Could you check a few things on this model? Use its own coordinates, in mm. Face numbers are marked on the shaded views. A direction names the side the tool comes from. Round coordinates to 2 decimals unless told otherwise and drop trailing zeros. Loops run counter-clockwise (first coordinate to the right, second up) from the corner with the lowest first, then second, coordinate; pieces in that order, holes last. Notation, with made-up numbers: (-35.5, -30) -> (-25.5, -30) arc R14 cw to (-25.5, -12) -> close; hole circle Ø1 at (-23, 22). An arc over 180 degrees is marked (long way). Write each question's results on one line, items separated by ' | '.
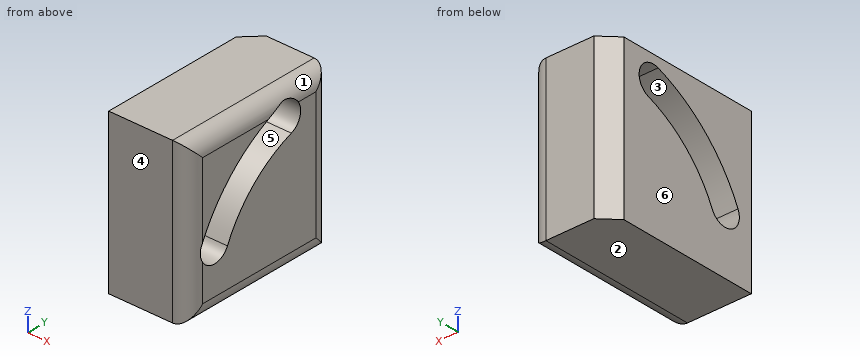
from build123d import *

# Parameters (mm, degrees)
F0_W     = 10
F0_H     = 20
F1_DEPTH = 20
F2_R     = 2
F3_SIZE  = 2
F5_DEPTH = 24.4


with BuildPart() as f1:
    # F0 (on Front) → F1 (new body)
    with BuildSketch(Plane.XZ):
        with Locations((5, 10)):
            Rectangle(F0_W, F0_H)
    extrude(amount=F1_DEPTH)

    # F2
    f2_edges = [f1.edges().sort_by_distance(p)[0] for p in [
        (10, -10, 0),
        (10, -10, 20),
        (10, 0, 10),
        (10, -20, 10),
    ]]
    fillet(f2_edges, radius=F2_R)

    # F3
    f3_edges = [f1.edges().sort_by_distance(p)[0] for p in [
        (0, 0, 10),
    ]]
    chamfer(f3_edges, length=F3_SIZE)

    # F4 (on face) → F5 (cut)
    with BuildSketch(Plane.YZ.offset(10)):
        with BuildLine():
            ThreePointArc((-5.472322, 15.035082), (-4.276977, 17.598507), (-6.840403, 18.793852))
            ThreePointArc((-6.840403, 18.793852), (-13.511804, 14.745547), (-18.126156, 8.452365))
            ThreePointArc((-18.126156, 8.452365), (-17.158777, 5.794513), (-14.500925, 6.761892))
            ThreePointArc((-14.500925, 6.761892), (-10.809443, 11.796437), (-5.472322, 15.035082))
        make_face()
    extrude(amount=-F5_DEPTH, mode=Mode.SUBTRACT)


solid = f1.part
1) For the marked faces 5 and 6, which set-ups out of +Z, -Z, +X, -X, +Y, -Y let a thin tool reach every point of the face, with its end or its side?
Model answer:
face 5: +X, -X | face 6: +Z, -Z, -X, +Y, -Y
2) I want a section at D-D, the plane y = -13.25. Write out the boundary of the cut face in (x, z), plus the area to 3 significant figures.
Model answer:
outline: (0, 0) -> (8, 0) arc R2 ccw to (10, 2) -> (10, 8.97) -> (0, 8.97) -> close; (0, 14.98) -> (10, 14.98) -> (10, 18) arc R2 ccw to (8, 20) -> (0, 20) -> close | area: 138 mm2
3) I need wall thicknesses on line 1 (Y direction, x = 3, z = 6.75); line 2 (Z direction, x = 3.5, y = -8.5); line 3 (Z direction, x = 4.75, y = -10.25). Which ranges of each line are inside material? Lowest first, please.
Model answer:
line 1: y = -20 to -18.12, -14.51 to 0 | line 2: z = 0 to 13.56, 18.1 to 20 | line 3: z = 0 to 12.29, 17.17 to 20
4) I want a section at B-B, the plane z = 14. Write out the boundary of the cut face in (x, y).
Model answer:
outline: (0, -20) -> (8, -20) arc R2 ccw to (10, -18) -> (10, -14.28) -> (0, -14.28) -> close; (0, -7.75) -> (10, -7.75) -> (10, -2) arc R2 ccw to (8, 0) -> (2, 0) -> (0, -2) -> close
5) I'm going to push a flat-ended pin straight in: pin 1 (1 mm diameter, centred on x = 8.5, y = -9.5, fed in from +Z). Where does the tip first touch, or does it pass through?
Model answer:
pin 1: stops at z = 20
6) I want a section at A-A, the plane y = -9.5. Write out the boundary of the cut face in (x, z), plus the area to 3 significant figures.
Model answer:
outline: (0, 0) -> (8, 0) arc R2 ccw to (10, 2) -> (10, 12.87) -> (0, 12.87) -> close; (0, 17.6) -> (10, 17.6) -> (10, 18) arc R2 ccw to (8, 20) -> (0, 20) -> close | area: 151 mm2
7) I want a section at C-C, the plane x = 7.5. Write out the boundary of the cut face in (y, z), plus the area to 3 significant figures.
Model answer:
outline: (-20, 0) -> (0, 0) -> (0, 20) -> (-20, 20) -> close; hole (-18.13, 8.45) arc R2 ccw to (-14.5, 6.76) arc R16 cw to (-5.47, 15.04) arc R2 ccw to (-6.84, 18.79) arc R20 ccw to start | area: 331 mm2
8) If we mould it in two halves opening along Z, with no side actions, what happens to the marked faces 1, 2, 3 and 4? For each: released by +Z, released by -Z, zero draft, split by the parting line, or undercut.
Model answer:
face 1: released by +Z | face 2: released by -Z | face 3: undercut | face 4: zero draft
